Input: part model. Units: mm. Frame: model coordinates. A direction names the side the tool comes from. Round coordinates to 2 decimals unless told otherwise and drop trailing zeros. Order: outer loops, then holes, each group sorted by start corner. A loop starts at its lowest first (then second) coordinate and runs counter-clockwise, first axis right, second up. Notation, with made-up numbers: (62.5, 65) -> (88.5, 65) arc R9 cw to (88.5, 77) -> close; hole circle Ø6 at (27.5, -17.5). An arc over 180 degrees is marked (long way). Use a Markdown table: item, result.
Autodesk Inventor part; units mm, degrees
ref_plane "YZ Plane" through (0, 0, 0) normal (1, 0, 0) x (0, 1, 0)
ref_plane "XZ Plane" through (0, 0, 0) normal (0, 1, 0) x (-1, 0, 0)
ref_plane "XY Plane" through (0, 0, 0) normal (0, 0, 1) x (1, 0, 0)
sketch "Sketch2" plane through (0, 0, 0) normal (0, 1, 0) x (-1, 0, 0)
  line L0 (0, 0) -> (60, 0)
  line L1 (60, 0) -> (60, -90)
  line L2 (60, -90) -> (0, -90)
  line L3 (0, -90) -> (0, 0)
  dimension "d5" = 60
  dimension "d6" = 90
extrude "Extrusion1" add sketch "Sketch2" along normal mid plane 10
sketch "Sketch3" plane through (0, 5, 0) normal (0, 1, 0) x (1, 0, 0)
  line L0 (-60, 0) -> (0, 0) construction
  line L1 (0, 0) -> (-31.8198, 31.8198) construction
  line L2 (0, 0) -> (45, 0) construction
  circle A0 centre (-31.8198, 31.8198) radius 12
  dimension "d9" = 45
  dimension "d10" = 135
  dimension "d11" = 24
extrude "Extrusion2" cut sketch "Sketch3" against normal blind 2
chamfer "Chamfer1" distance 10 angle 45 1 edges at (0, 0, 0)
fillet "Fillet1" radius 6 1 edges at (-60, 0, -90)
fillet "Fillet1" radius 2 4 edges at (-30, 5, -90) (-30, -5, -90) (-60, -5, -45) (-60, 5, -45)
sketch "Sketch4" plane through (0, 5, 0) normal (0, 1, 0) x (1, 0, 0)
  circle A0 centre (-31.8198, 31.8198) radius 12
  line L0 (-31.8198, 31.8198) -> (-12.8198, 31.8198) construction
  line L1 (-12.8198, 31.8198) -> (-12.8198, 20.8198) construction
  circle A1 centre (-12.8198, 20.8198) radius 2
  line L2 (-31.8198, 31.8198) -> (-31.8198, 62.8198) construction
  line L3 (-31.8198, 31.8198) -> (-31.8198, 76.8198) construction
  circle A2 centre (-50.8198, 20.8198) radius 2
  line L4 (-31.8198, 76.8198) -> (-12.8198, 76.8198) construction
  line L5 (-31.8198, 62.8198) -> (-50.8198, 62.8198) construction
  circle A3 centre (-12.8198, 76.8198) radius 2
  circle A4 centre (-50.8198, 62.8198) radius 2
  point P0 (0, 0)
  dimension "d19" = 19
  dimension "d20" = 11
  dimension "d21" = 4
  dimension "d22" = 31
  dimension "d30" = 19
  dimension "d32" = 19
  dimension "d33" = 45
  dimension "d34" = 4
  dimension "d35" = 4
extrude "Extrusion4" cut sketch "Sketch4" against normal up to surface (10 mm away) contours A1 | A2 | A3 | A4
sketch "Sketch6" plane through (0, -5, 0) normal (0, -1, 0) x (1, 0, 0)
  circle A0 centre (-50.8198, -20.8198) radius 2
  circle A1 centre (-12.8198, -20.8198) radius 2
  circle A2 centre (-50.8198, -62.8198) radius 2
  circle A3 centre (-12.8198, -76.8198) radius 2
  circle A4 centre (-50.8198, -20.8198) radius 2
  circle A5 centre (-50.8198, -20.8198) radius 4.5
  circle A6 centre (-12.8198, -20.8198) radius 2
  circle A7 centre (-12.8198, -20.8198) radius 4.5
  circle A8 centre (-50.8198, -62.8198) radius 4.5
  circle A9 centre (-12.8198, -76.8198) radius 2
  circle A10 centre (-12.8198, -76.8198) radius 4.5
  point P0 (0, 0)
  dimension "d45" = 9
  dimension "d46" = 9
  dimension "d47" = 9
  dimension "d48" = 9
extrude "Extrusion6" cut sketch "Sketch6" against normal blind 4
sketch "Sketch7" plane through (0, 5, 0) normal (0, 1, 0) x (1, 0, 0)
  circle A0 centre (-12.8198, 20.8198) radius 2
  circle A1 centre (-50.8198, 20.8198) radius 2
  circle A2 centre (-50.8198, 62.8198) radius 2
  circle A3 centre (-12.8198, 76.8198) radius 2
  circle A4 centre (-12.8198, 20.8198) radius 2
  circle A5 centre (-12.8198, 20.8198) radius 5
  circle A6 centre (-50.8198, 20.8198) radius 5
  circle A7 centre (-12.8198, 76.8198) radius 5
  circle A8 centre (-50.8198, 62.8198) radius 5
  point P0 (0, 0)
  dimension "d51" = 10
  dimension "d52" = 10
  dimension "d53" = 10
  dimension "d54" = 10
extrude "Extrusion7" cut sketch "Sketch7" against normal blind 1
thread "Thread1"
thread "Thread2"
thread "Thread3"
thread "Thread4"
properties part number "bearing bracket for bolt screw"
1) Pin query (flat end, axial travel): pin 1 Ø2.5 at (x, z) = (-50.82, -20.82) entering from -Y; pin 2 Ø5 at (x, z) = (-52, -19) entering from +Y; pin 3 Ø2.5 at (x, z) = (-11.5, -18.5) entering from -Y. Return the tip coordinate at first contact, or that it passes through.
Results found:
| item | result |
|---|---|
| pin 1 | passes through |
| pin 2 | stops at y = 4 |
| pin 3 | stops at y = -1 |
2) Cut plane B-B on x = -36. Return loops of the section in (y, z).
Results found:
| item | result |
|---|---|
| outline | (-5, -88) arc R2 ccw to (-3, -90) -> (3, -90) arc R2 ccw to (5, -88) -> (5, -43.07) -> (3, -43.07) -> (3, -20.57) -> (5, -20.57) -> (5, 0) -> (-5, 0) -> close |
3) Cut plane C-C on y = 0. Return loops of the section in (x, z).
Results found:
| item | result |
|---|---|
| outline | (-60, -84) arc R6 ccw to (-54, -90) -> (0, -90) -> (0, -10) -> (-10, 0) -> (-60, 0) -> close; hole circle Ø4 at (-50.82, -62.82); hole circle Ø4 at (-50.82, -20.82); hole circle Ø4 at (-12.82, -76.82); hole circle Ø4 at (-12.82, -20.82) |
4) Cut plane D-D on x = -25. Return loops of the section in (y, z), and give its area (3 significant figures).
Results found:
| item | result |
|---|---|
| outline | (-5, -88) arc R2 ccw to (-3, -90) -> (3, -90) arc R2 ccw to (5, -88) -> (5, -41.69) -> (3, -41.69) -> (3, -21.95) -> (5, -21.95) -> (5, 0) -> (-5, 0) -> close |
| area | 859 mm² |
5) Set-up query: faces 4 (the flat face through (-10.67, 4, -76.89)), 5 (the cylindrical face through (-14.407, 1.535, -19.603)), 6 (the cylindrical face through (-13.41, -3.03, -72.36)). Return all of +Z, -Z, +X, -X, +Y, -Y with unobstructed straight access to the full face (end or side cutting, diameter ignored); none if empty.
Results found:
| item | result |
|---|---|
| face 4 | +Y |
| face 5 | +Y, -Y |
| face 6 | -Y |
6) Cut plane A-A on z = -8. Return loops of the section in (x, y).
Results found:
| item | result |
|---|---|
| outline | (-60, -3) arc R2 ccw to (-58, -5) -> (-2, -5) -> (-2, 5) -> (-58, 5) arc R2 ccw to (-60, 3) -> close |
7) Pull-direction query (X, two-part tool) for faces 1 (the flat face through (-27, 0, -90)), 2 (the cylindrical face through (-58.289, -0.042, -88.196)), 3 (the cylindrical face through (-51.471, 4.507, -67.777)); classes: +X half, -X half, draft (parallel to the pull), parting line (faces both ways), or undercut.
Results found:
| item | result |
|---|---|
| face 1 | draft |
| face 2 | -X half |
| face 3 | undercut |
8) Line query: L1, parallel to Z at x = -51, y = -0.5; L2, parallel to X at y = -4.5, z = -22.5; L3, parallel to Z at x = -17, y = 4.25. Output: solid intervals per line, ascending. Write a range as [from, to].
Results found:
| item | result |
|---|---|
| L1 | z = [-90, -64.81], [-60.83, -22.81], [-18.83, 0] |
| L2 | x = [-59.32, -54.99], [-46.65, -16.99], [-8.65, 0] |
| L3 | z = [-89.56, -79.56], [-74.08, -23.56], [-18.08, 0] |
